Verification items for the finished model (mm, model axes). A direction names the side the tool comes from. Coordinates: 2 decimals unless noted, no trailing zeros. Order: outer loops, then holes, each group sorted by start corner. A loop starts at its lowest first (then second) coordinate and runs counter-clockwise, first axis right, second up. Notation, with made-up numbers: M -20.5,71.25 L 10.5,71.25 A13 cw 10.5,77.25 Z; hole C -16.75,41 d9. An arc over 180 degrees is marked long. Return JSON: item names as keys, results as strings. Group by question number.
Q1. Section check C-C, the plane z = 12.5. Enter the section's corners in (x, y), then the cut area to 3 significant figures.
Q2. Section check A-A, the plane x = 0. Enter the section's corners in (y, z), then the cut area to 3 significant figures.
Q3. Thickness scan on probe 1 along Z at (x, y) = (19, 9); probe 2 along X at (y, z) = (6.5, 19); probe 3 along X at (y, z) = (19, 27). Record the ranges inside material, lowest first.
Q4. Go/stop test with flat-tipped pins: pin 1 Ø3 at (x, z) = (9.5, 16) entering from +Y; pin 2 Ø1.5 at (x, y) = (-22, 6) entering from -Z; pin 3 Ø8 at (y, z) = (1, 8.5) entering from -X. Record where each tip stops, or that it passes through.
Q5. Access from +Z, -Z, +X, -X, +Y, -Y to the whole of each face (thin tool, end or side, straight path). Record for faces 1 (the face through (11.37, -2.53, 10.63)), 2 (the face through (0, 0, 30)).
from build123d import *


with BuildPart() as f1:
    # F0 (on Right) → F1 (revolve)
    with BuildSketch(Plane.YZ):
        with BuildLine():
            Line((0, 30), (0, 0))
            Line((0, 0), (10.65, 0))
            ThreePointArc((10.65, 0), (11.357107, 0.292893), (11.65, 1))
            Line((11.65, 1), (11.65, 20))
            Line((11.65, 20), (28, 20))
            ThreePointArc((28, 20), (29.414214, 20.585786), (30, 22))
            Line((30, 22), (30, 24))
            ThreePointArc((30, 24), (28.242641, 28.242641), (24, 30))
            Line((24, 30), (0, 30))
        make_face()
    revolve(axis=Axis((0, 0, 15), (0, 0, 1)))


solid = f1.part
Numbers:
{
 "1": {"outline": "C 0,0 d23.3", "area": "426 mm2"},
 "2": {"outline": "M -30,22 A2 ccw -28,20 L -11.65,20 L -11.65,1 A1 ccw -10.65,0 L 10.65,0 A1 ccw 11.65,1 L 11.65,20 L 28,20 A2 ccw 30,22 L 30,24 A6 ccw 24,30 L -24,30 A6 ccw -30,24 Z", "area": "1,050 mm2"},
 "3": {"probe 1": "z = 20 to 30", "probe 2": "x = -9.67 to 9.67", "probe 3": "x = -22.17 to 22.17"},
 "4": {"pin 1": "stops at y = 8.47", "pin 2": "stops at z = 20", "pin 3": "stops at x = -11.65"},
 "5": {"face 1": "-Z", "face 2": "+Z, +X, -X, +Y, -Y"}
}
